Source: CAD feature listing. Evaluate the final solid. Frame: model axes, mm. Give positions to 0.01 mm unless a question says otherwise; leave off trailing zeros. Order: outer loops, then holes, each group sorted by start corner. A loop starts at its lowest first (then second) coordinate and runs counter-clockwise, first axis right, second up. Notation, with made-up numbers: M 21.25,25.25 L 31.25,25.25 A9 cw 31.25,36.25 Z; hole C 12.25,1.5 d2. An arc over 180 degrees is marked long. Use CSV: the item, a comma, the result in double quotes. Start each with the question number.
1. Section query C-C, the plane x = 0. Return the cut outline in (y, z), plus the area to 3 significant figures.
2. Section query D-D, the plane z = 172. Return the cut outline in (x, y).
3. Section query B-B, the plane z = 5. State how many separate pieces and enclosed holes the cut face has, plus the area to 3 significant figures.
4. Line query: line 1 along Y through (x, z) = (0, 5); line 2 along X through (y, z) = (-1, 172); line 3 along Z through (x, y) = (-25, -2). Output: solid intervals per line, ascending. Write a range as [from, to].
5. Pin query (flat end, axial travel): P1, Ø6.5, axis at x = -21.5, z = 5.5, coming from the +Y side; P2, Ø12, axis at y = 5.5, z = 60, coming from the +X side; P3, Ø8, axis at y = 17, z = 3, coming from the -X side; P4, Ø4.5, axis at x = 0, y = 0, coming from the +Z side. Return the tip coordinate at first contact, or that it passes through.
6. Section query A-A, the plane x = 10. Return the cut outline in (y, z).
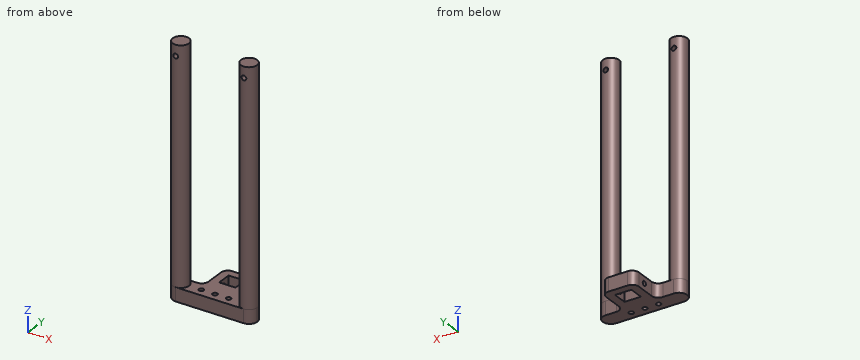
from build123d import *

# Parameters (mm, degrees)
SKETCH1_W               = 62
SKETCH1_H               = 12
BOSS_EXTRUDE1_DEPTH     = 10
SKETCH2_R               = 6
BOSS_EXTRUDE2_DEPTH     = 170
SKETCH3_W               = 24
SKETCH3_H               = 10
BOSS_EXTRUDE3_DEPTH     = 24
CUT_EXTRUDE1_REACH      = 187.097
SKETCH4_W               = 12
SKETCH4_H               = 10.5
SKETCH5_R               = 1.75
CUT_EXTRUDE2_DEPTH      = 188.48066567
FILLET1_R               = 6
FILLET2_R               = 5
CUT_EXTRUDE3_DEPTH      = 186.097271725
CUT_EXTRUDE3_DEPTH_BACK = 186.097271725
SKETCH6_R               = 1.75
CUT_EXTRUDE4_REACH      = 187.097
SKETCH7_R               = 1.75
CUT_EXTRUDE5_REACH      = 187.097
SKETCH8_R               = 1.75


with BuildPart() as part:
    # Sketch1 → Boss-Extrude1 (new body)
    with BuildSketch(Plane.XY):
        Rectangle(SKETCH1_W, SKETCH1_H)
    extrude(amount=BOSS_EXTRUDE1_DEPTH)

    # Sketch2 → Boss-Extrude2 (add)
    with BuildSketch(Plane.XY.offset(10)):
        with Locations(Location((-25, 0, 0), (0, 0, 180))):
            Circle(SKETCH2_R)
        with Locations((25, 0)):
            Circle(SKETCH2_R)
    extrude(amount=BOSS_EXTRUDE2_DEPTH)

    # Sketch3 → Boss-Extrude3 (add)
    with BuildSketch(Plane(origin=(0, 6, 0), x_dir=(1, 0, 0), z_dir=(0, 1, 0))):
        with Locations((0, -5)):
            Rectangle(SKETCH3_W, SKETCH3_H)
    extrude(amount=BOSS_EXTRUDE3_DEPTH)

    # Sketch4 → Cut-Extrude1 (cut, up to next)
    with BuildSketch(Plane(origin=(0, 0, 0), x_dir=(-1, 0, 0), z_dir=(0, 0, -1)), mode=Mode.PRIVATE) as cut_extrude1_sk1:
        with Locations((0, 19)):
            Rectangle(SKETCH4_W, SKETCH4_H)
    cut_extrude1_tool1 = extrude(cut_extrude1_sk1.sketch, amount=-CUT_EXTRUDE1_REACH, mode=Mode.PRIVATE) & part.part
    add(cut_extrude1_tool1.solids().sort_by_distance((0, 19, 0))[0], mode=Mode.SUBTRACT)

    # Sketch5 → Cut-Extrude2 (cut, through all)
    with BuildSketch(Plane(origin=(12, 0, 0), x_dir=(0, 0, -1), z_dir=(1, 0, 0))):
        with Locations((-5, 19)):
            Circle(SKETCH5_R)
    extrude(amount=-CUT_EXTRUDE2_DEPTH, mode=Mode.SUBTRACT)

    # Fillet1
    fillet1_edges = [part.edges().sort_by_distance(p)[0] for p in [
        (-31, -6, 5),
        (-31, 6, 5),
        (31, 6, 5),
        (31, -6, 5),
    ]]
    fillet(fillet1_edges, radius=FILLET1_R - 0.0001)  # a hair under: the kernel refuses the full size

    # Fillet2
    fillet2_edges = [part.edges().sort_by_distance(p)[0] for p in [
        (-12, 6, 5),
        (12, 6, 5),
        (-12, 30, 5),
        (12, 30, 5),
    ]]
    fillet(fillet2_edges, radius=FILLET2_R)

    # Sketch6 → Cut-Extrude3 (cut, two sides: drawn at the far end of the back side and taken through both)
    with BuildSketch(Plane(origin=(0, 0, 0), x_dir=(1, 0, 0), z_dir=(0, 1, 0)).offset(-CUT_EXTRUDE3_DEPTH_BACK)):
        with Locations(Location((-25, -172, 0), (0, 0, 270))):
            Circle(SKETCH6_R)
        with Locations(Location((25, -172, 0), (0, 0, 270))):
            Circle(SKETCH6_R)
    extrude(amount=CUT_EXTRUDE3_DEPTH + CUT_EXTRUDE3_DEPTH_BACK, mode=Mode.SUBTRACT)

    # Sketch7 → Cut-Extrude4 (cut, up to next)
    with BuildSketch(Plane(origin=(0, 0, 0), x_dir=(-1, 0, 0), z_dir=(0, 0, -1)), mode=Mode.PRIVATE) as cut_extrude4_sk1:
        with Locations((-10, 0)):
            Circle(SKETCH7_R)
    cut_extrude4_tool1 = extrude(cut_extrude4_sk1.sketch, amount=-CUT_EXTRUDE4_REACH, mode=Mode.PRIVATE) & part.part
    # Sketch7 → Cut-Extrude4 (cut, up to next)
    with BuildSketch(Plane(origin=(0, 0, 0), x_dir=(-1, 0, 0), z_dir=(0, 0, -1)), mode=Mode.PRIVATE) as cut_extrude4_sk2:
        with Locations((10, 0)):
            Circle(SKETCH7_R)
    cut_extrude4_tool2 = extrude(cut_extrude4_sk2.sketch, amount=-CUT_EXTRUDE4_REACH, mode=Mode.PRIVATE) & part.part
    add(cut_extrude4_tool1.solids().sort_by_distance((10, 0, 0))[0], mode=Mode.SUBTRACT)
    add(cut_extrude4_tool2.solids().sort_by_distance((-10, 0, 0))[0], mode=Mode.SUBTRACT)

    # Sketch8 → Cut-Extrude5 (cut, up to next)
    with BuildSketch(Plane(origin=(0, 0, 0), x_dir=(-1, 0, 0), z_dir=(0, 0, -1)), mode=Mode.PRIVATE) as cut_extrude5_sk1:
        Circle(SKETCH8_R)
    cut_extrude5_tool1 = extrude(cut_extrude5_sk1.sketch, amount=-CUT_EXTRUDE5_REACH, mode=Mode.PRIVATE) & part.part
    add(cut_extrude5_tool1.solids().sort_by_distance((0, 0, 0))[0], mode=Mode.SUBTRACT)


solid = part.part
Result set:
1,outline,"M -6,0 L -1.75,0 L -1.75,10 L -6,10 Z; M 1.75,0 L 13.75,0 L 13.75,10 L 1.75,10 Z; M 24.25,0 L 30,0 L 30,10 L 24.25,10 Z"
1,area,"220 mm2"
2,outline,"M -26.75,-5.74 L -26.75,5.74 A6 ccw Z; M -23.25,-5.74 A6 ccw -23.25,5.74 Z; M 23.25,-5.74 L 23.25,5.74 A6 ccw Z; M 26.75,-5.74 A6 ccw 26.75,5.74 Z"
3,separate pieces,"2"
3,enclosed holes,"3"
3,area,"1,090 mm2"
4,line 1,"[-6, -1.75], [1.75, 13.75], [24.25, 30]"
4,line 2,"[-30.92, -26.75], [-23.25, -19.08], [19.08, 23.25], [26.75, 30.92]"
4,line 3,"[0, 170.25], [173.75, 180]"
5,P1,"y = 6"
5,P2,"x = 31"
5,P3,"x = -12"
5,P4,"z = 10"
6,outline,"M -6,0 L -1.75,0 L -1.75,10 L -6,10 Z; M 1.75,0 L 29,0 L 29,10 L 1.75,10 Z; hole C 19,5 d3.5"
